Drawing for the job (mm, zero at the part's lowest x, y, z). A direction names the side the tool comes from. Coordinates: 2 decimals unless noted, no trailing zeros. Order: outer loops, then holes, each group sorted by start corner. A loop starts at its lowest first (then second) coordinate and runs counter-clockwise, first axis right, second up. Notation, with made-up numbers: (-15, 88.25) -> (0, 88.25) arc R11 ccw to (0, 97.25) -> close; hole circle Ø9 at (86, -3.5). An arc over 180 degrees is marked (long way). Write each question's results on one line, items separated by ' | '.
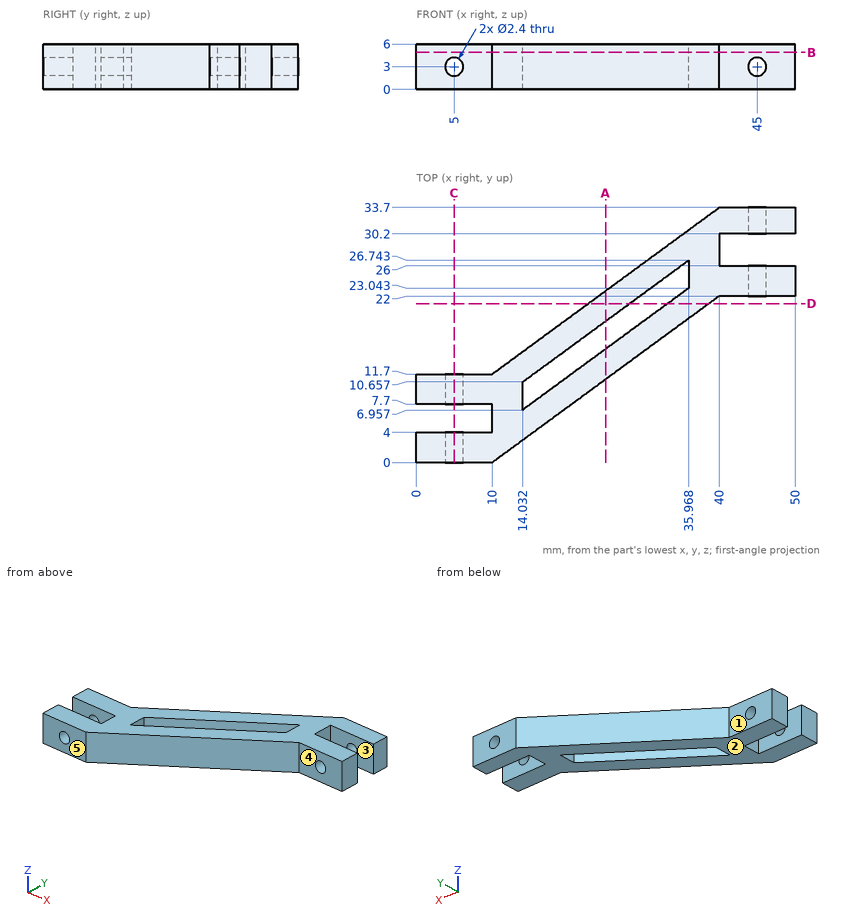
Item 1: Slice it at A-A, the plane x = 25. List the corners of the cut face in (y, z).
Answer:
outline: (11, 0) -> (15, 0) -> (15, 6) -> (11, 6) -> close; (18.7, 0) -> (22.7, 0) -> (22.7, 6) -> (18.7, 6) -> close
Item 2: Pull direction Y, two halves, no side cores. Call the marked faces 1, 2 and 3: released by +Y, released by -Y, zero draft, split by the parting line, or undercut.
Answer:
face 1: released by +Y | face 2: zero draft | face 3: undercut
Item 3: Drill centre lines: line 1 (Y direction, x = 46.5, z = 5.35); line 2 (Z direction, x = 5, y = 10.6); line 3 (Y direction, x = 19, z = 4.5). Where is each one in solid material? Low to high. Write a range as from..to.
Answer:
line 1: y = 22..26, 30.2..33.7 | line 2: z = 0..1.8, 4.2..6 | line 3: y = 6.6..10.6, 14.3..18.3
Item 4: Pin check, flat tips, straight feed: pin 1 (2 mm diameter, centred on x = 45, z = 3, fed in from -Y); pin 2 (3 mm diameter, centred on x = 46, z = 2.5, fed in from -Y); pin 3 (1 mm diameter, centred on y = 16.5, z = 1.5, fed in from +X); pin 4 (2 mm diameter, centred on x = 19.5, z = 1, fed in from +Y). Stop position of each tip, or through.
Answer:
pin 1: passes through | pin 2: stops at y = 22 | pin 3: stops at x = 33.18 | pin 4: stops at y = 19.4
Item 5: Slice it at D-D, the plane y = 21. List the corners of the cut face in (x, z).
Answer:
outline: (22.68, 0) -> (28.14, 0) -> (28.14, 6) -> (22.68, 6) -> close; (33.18, 0) -> (38.64, 0) -> (38.64, 6) -> (33.18, 6) -> close
Item 6: Slice it at B-B, the plane z = 4.9. List the corners of the cut face in (x, y), and give its area (3 significant figures).
Answer:
outline: (0, 0) -> (10, 0) -> (40, 22) -> (50, 22) -> (50, 26) -> (40, 26) -> (40, 30.2) -> (50, 30.2) -> (50, 33.7) -> (40, 33.7) -> (10, 11.7) -> (0, 11.7) -> (0, 7.7) -> (10, 7.7) -> (10, 4) -> (0, 4) -> close; hole (14.03, 6.96) -> (35.97, 23.04) -> (35.97, 26.74) -> (14.03, 10.66) -> close | area: 425 mm^2
Item 7: Slice it at C-C, the plane x = 5. List the corners of the cut face in (y, z).
Answer:
outline: (0, 0) -> (4, 0) -> (4, 1.8) -> (0, 1.8) -> close; (0, 4.2) -> (4, 4.2) -> (4, 6) -> (0, 6) -> close; (7.7, 0) -> (11.7, 0) -> (11.7, 1.8) -> (7.7, 1.8) -> close; (7.7, 4.2) -> (11.7, 4.2) -> (11.7, 6) -> (7.7, 6) -> close
Item 8: Tool access for the marked faces 4 and 5: list every direction of +Z, -Z, +X, -X, +Y, -Y with a clear straight run to the whole face (end or side of a thin tool).
Answer:
face 4: +Z, -Z, +X, -Y | face 5: +Z, -Z, +X, -X, -Y
